```python
from build123d import *

# Parameters (mm, degrees)
CROQUIS1_R              = 60
SALIENTE_EXTRUIR3_DEPTH = 25
CROQUIS4_W              = 100
CROQUIS4_H              = 3
SALIENTE_EXTRUIR5_DEPTH = 150
CORTAR_EXTRUIR3_DEPTH   = 150
CROQUIS11_R             = 3
CORTAR_EXTRUIR4_DEPTH   = 150


with BuildPart() as part:
    # Croquis1 → Saliente-Extruir3 (new body)
    with BuildSketch(Plane(origin=(0, 0, 0), x_dir=(1, 0, 0), z_dir=(0, 1, 0))):
        Circle(CROQUIS1_R)
    extrude(amount=SALIENTE_EXTRUIR3_DEPTH)

    # Croquis4 → Saliente-Extruir5 (add)
    with BuildSketch(Plane(origin=(0, 25, 0), x_dir=(1, 0, 0), z_dir=(0, 1, 0))):
        with Locations((0, 16.5)):
            Rectangle(CROQUIS4_W, CROQUIS4_H)
        Polygon((0, -15), (50, -15), (50, -18), (-50, -18), (-50, -15), align=None)
    extrude(amount=SALIENTE_EXTRUIR5_DEPTH)

    # Croquis10 → Cortar-Extruir3 (cut)
    with BuildSketch(Plane.XY.offset(18)):
        Polygon((-50, 175), (-15, 175), (-50, 25), align=None)
        Polygon((50, 25), (15, 175), (50, 175), align=None)
    extrude(amount=-CORTAR_EXTRUIR3_DEPTH, mode=Mode.SUBTRACT)

    # Croquis11 → Cortar-Extruir4 (cut)
    with BuildSketch(Plane.XY.offset(18)):
        with Locations((0, 160)):
            Circle(CROQUIS11_R)
    extrude(amount=-CORTAR_EXTRUIR4_DEPTH, mode=Mode.SUBTRACT)


solid = part.part
```
The model under review builds one solid part; all positions refer to its coordinate system, in mm. A direction names the side the tool comes from. Coordinates: 2 decimals unless noted, no trailing zeros. Write each loop counter-clockwise with the first axis right and the second up, starting at its lowest first coordinate (ties: lowest second). Pieces come first, ordered by that corner, then holes. Notation, with made-up numbers: (77, -34) -> (92, -34) arc R6 cw to (92, -23) -> close; hole circle Ø7 at (-21, 31). An arc over 180 degrees is marked (long way). One line per item, written item: value. Start each with the question number.
Q1. Add section B-B, the plane x = 0. Give the boundary of the cut face in (y, z).
Q2. Clearance check with flat-ended pins moving along their axes: P1, Ø5, axis at x = 0, y = 160, coming from the -Z side; P2, Ø1, axis at x = 20, y = 46, coming from the +Z side; P3, Ø8, axis at x = 27, y = 31.5, coming from the -Z side. State where each tip first meets the part, or that it passes through.
Q3. Add section D-D, the plane x = -39. Give the boundary of the cut face in (y, z), then the cut area to 3 significant figures.
Q4. The part is to be moulded in two halves that separate along Y. For faces 1 (the face through (-1, 82, -15)), 2 (the face through (1.61, 162.53, 16.52)), 3 (the face through (1.61, 162.53, -16.48)), 4 (the face through (-32.255, 101.05, 16.521)), say which applies: +Y half, -Y half, draft (parallel to the pull), parting line (faces both ways), or undercut.
Q5. To check wall thickness, follow probe 1 along Y at (x, z) = (0, -16.6); probe 2 along Z at (x, y) = (-15.5, 36); probe 3 along X at (y, z) = (160, 16). State the ranges of each line that lie inside material, in increasing order.
Q6. Add section C-C, the plane y = 64. Give the boundary of the cut face in (x, z).
Q7. Add section A-A, the plane y = 160. Give the boundary of the cut face in (x, z), then the cut area to 3 significant figures.
Q8. For faces 5 (the face through (1, 82, 18)), 6 (the face through (32.745, 98.95, -16.479)), 7 (the face through (1, 82, 15)), 8 (the face through (-1, 82, -18)), list the 3-axis set-ups (+Z, -Z, +X, -X, +Y, -Y) from which the entire face can be reached by the end or side of a thin tool; tool diameter is ignored.
Response:
1. outline: (0, -60) -> (25, -60) -> (25, -18) -> (157, -18) -> (157, -15) -> (25, -15) -> (25, 15) -> (157, 15) -> (157, 18) -> (25, 18) -> (25, 60) -> (0, 60) -> close; (163, -18) -> (175, -18) -> (175, -15) -> (163, -15) -> close; (163, 15) -> (175, 15) -> (175, 18) -> (163, 18) -> close
2. P1: through
2. P2: z = 18
2. P3: z = -18
3. outline: (0, -45.6) -> (25, -45.6) -> (25, -18) -> (72.14, -18) -> (72.14, -15) -> (25, -15) -> (25, 15) -> (72.14, 15) -> (72.14, 18) -> (25, 18) -> (25, 45.6) -> (0, 45.6) -> close
3. area: 2,560 mm²
4. face 1: draft
4. face 2: undercut
4. face 3: undercut
4. face 4: +Y half
5. probe 1: 0 to 157, 163 to 175
5. probe 2: -18 to -15, 15 to 18
5. probe 3: -18.5 to -3, 3 to 18.5
6. outline: (-40.9, -18) -> (40.9, -18) -> (40.9, -15) -> (-40.9, -15) -> close; (-40.9, 15) -> (40.9, 15) -> (40.9, 18) -> (-40.9, 18) -> close
7. outline: (-18.5, -18) -> (-3, -18) -> (-3, -15) -> (-18.5, -15) -> close; (-18.5, 15) -> (-3, 15) -> (-3, 18) -> (-18.5, 18) -> close; (3, -18) -> (18.5, -18) -> (18.5, -15) -> (3, -15) -> close; (3, 15) -> (18.5, 15) -> (18.5, 18) -> (3, 18) -> close
7. area: 186 mm²
8. face 5: +Z, +X, -X, +Y
8. face 6: +Z, -Z, +X, +Y
8. face 7: +X, -X, +Y
8. face 8: -Z, +X, -X, +Y
